Study the drawing (mm; zero at the part's minimum x, y, z) and answer. Round coordinates to 2 decimals unless told otherwise and drop trailing zeros. Write each loop counter-clockwise with the first axis right and the second up, starting at its lowest first coordinate (ties: lowest second). Pieces come first, ordered by that corner, then holes. Notation, with made-up numbers: (8.5, -2.5) -> (18.5, -2.5) arc R21 cw to (18.5, 26.5) -> close; hole circle Ø6 at (-23, -36.75). An arc over 180 degrees is marked (long way). One line per question, with ' | ' between items. Start each with the question number.
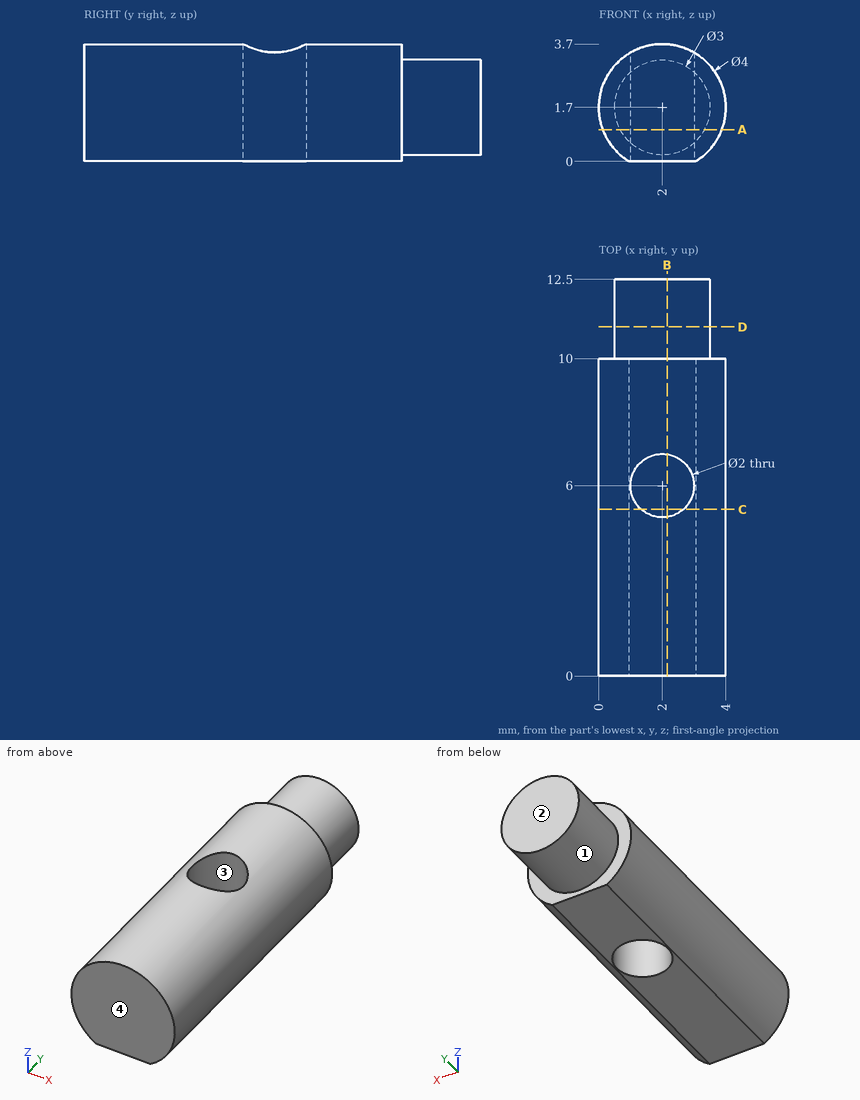
(1) A cutting plane is placed at D-D, the plane y = 11. Determine the outline of the cut face in (x, z).
(2) A cutting plane is placed at A-A, the plane z = 1. Determine the outline of the cut face in (x, y).
(3) Given pin 1 Ø2 at (x, y) = (0.5, 5) entering from +Z; pin 2 Ø1 at (y, z) = (2.5, 1.5) entering from +X, each flat-ended and moving along its own axis, determine where each tip first touches the part or whether it passes through.
(4) Consider L1, parallel to Y at x = 2, z = 1.9; L2, parallel to X at y = 11.5, z = 1.6; L3, parallel to Z at x = 2.05, y = 11.75. Determine where each line is inside the solid, lowest interval first.
(5) A cutting plane is placed at B-B, the plane x = 2.15. Determine the outline of the cut face in (y, z), then the cut area to 3 significant figures.
(6) A cutting plane is placed at C-C, the plane y = 5.25. Determine the outline of the cut face in (x, z).
(7) The mould has two halves that part along Y. Classify the marked faces 1, 2, 3 and 4: +Y half, -Y half, draft (parallel to the pull), parting line (faces both ways), or undercut.
Returned:
1) outline: circle Ø3 at (2, 1.7)
2) outline: (0.13, 0) -> (3.87, 0) -> (3.87, 10) -> (3.33, 10) -> (3.33, 12.5) -> (0.67, 12.5) -> (0.67, 10) -> (0.13, 10) -> close; hole circle Ø2 at (2, 6)
3) pin 1: z = 3.64 | pin 2: x = 4
4) L1: 0 to 5, 7 to 12.5 | L2: 0.5 to 3.5 | L3: 0.2 to 3.2
5) outline: (0, 0) -> (5.01, 0) -> (5.01, 3.69) -> (0, 3.69) -> close; (6.99, 0) -> (10, 0) -> (10, 0.21) -> (12.5, 0.21) -> (12.5, 3.19) -> (10, 3.19) -> (10, 3.69) -> (6.99, 3.69) -> close | area: 37.1 mm2
6) outline: (0.95, 0) -> (1.34, 0) -> (1.34, 3.59) arc R2 ccw to start; (2.66, 0) -> (3.05, 0) arc R2 ccw to (2.66, 3.59) -> close
7) face 1: draft | face 2: +Y half | face 3: undercut | face 4: -Y half
